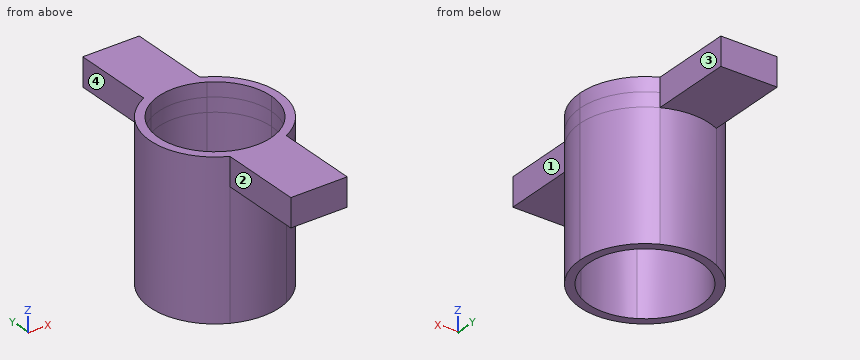
from build123d import *

# Parameters (mm, degrees)
F1_DEPTH = 10
F2_DEPTH = 1


# Not quite as in the source:
# - a feature names something its author has since deleted; it is built from what else it names


with BuildPart() as f1:
    # F0 (on Top) → F1 (new body)
    with BuildSketch(Plane.XY):
        with BuildLine():
            Line((-2, 3.4641016151), (-2, 4.1424630354))
            ThreePointArc((-2, 4.1424630354), (-4.6, 0), (-2, -4.1424630354))
            Line((-2, -4.1424630354), (-2, -3.4641016151))
            ThreePointArc((-2, -3.4641016151), (-4, 0), (-2, 3.4641016151))
        make_face()
        with BuildLine():
            ThreePointArc((-2, -4.1424630354), (0, -4.6), (2, -4.1424630354))
            Line((2, -4.1424630354), (2, -3.4641016151))
            ThreePointArc((2, -3.4641016151), (0, -4), (-2, -3.4641016151))
            Line((-2, -3.4641016151), (-2, -4.1424630354))
        make_face()
        with BuildLine():
            ThreePointArc((2, -4.1424630354), (3.8961519478, -2.4454038521), (4.6, 0))
            ThreePointArc((4.6, 0), (3.8961519478, 2.4454038521), (2, 4.1424630354))
            Line((2, 4.1424630354), (2, 3.4641016151))
            ThreePointArc((2, 3.4641016151), (3.4641016151, 2), (4, 0))
            ThreePointArc((4, 0), (3.4641016151, -2), (2, -3.4641016151))
            Line((2, -3.4641016151), (2, -4.1424630354))
        make_face()
        with BuildLine():
            Line((2, 3.4641016151), (2, 4.1424630354))
            ThreePointArc((2, 4.1424630354), (0, 4.6), (-2, 4.1424630354))
            Line((-2, 4.1424630354), (-2, 3.4641016151))
            ThreePointArc((-2, 3.4641016151), (0, 4), (2, 3.4641016151))
        make_face()
    extrude(amount=-F1_DEPTH)

    # F0 (on Top) → F2 (join, symmetric)
    with BuildSketch(Plane.XY):
        with BuildLine():
            ThreePointArc((-2, 4.1424630354), (0, 4.6), (2, 4.1424630354))
            Line((2, 4.1424630354), (2, 10))
            Line((2, 10), (-2, 10))
            Line((-2, 10), (-2, 4.1424630354))
        make_face()
        with BuildLine():
            Line((2, -10), (2, -4.1424630354))
            ThreePointArc((2, -4.1424630354), (0, -4.6), (-2, -4.1424630354))
            Line((-2, -4.1424630354), (-2, -10))
            Line((-2, -10), (2, -10))
        make_face()
        with BuildLine():
            Line((2, 3.4641016151), (2, 4.1424630354))
            ThreePointArc((2, 4.1424630354), (0, 4.6), (-2, 4.1424630354))
            Line((-2, 4.1424630354), (-2, 3.4641016151))
            ThreePointArc((-2, 3.4641016151), (0, 4), (2, 3.4641016151))
        make_face()
        with BuildLine():
            ThreePointArc((-2, -4.1424630354), (0, -4.6), (2, -4.1424630354))
            Line((2, -4.1424630354), (2, -3.4641016151))
            ThreePointArc((2, -3.4641016151), (0, -4), (-2, -3.4641016151))
            Line((-2, -3.4641016151), (-2, -4.1424630354))
        make_face()
        with BuildLine():
            Line((-2, 3.4641016151), (-2, 4.1424630354))
            ThreePointArc((-2, 4.1424630354), (-4.6, 0), (-2, -4.1424630354))
            Line((-2, -4.1424630354), (-2, -3.4641016151))
            ThreePointArc((-2, -3.4641016151), (-4, 0), (-2, 3.4641016151))
        make_face()
        with BuildLine():
            ThreePointArc((2, -4.1424630354), (3.8961519478, -2.4454038521), (4.6, 0))
            ThreePointArc((4.6, 0), (3.8961519478, 2.4454038521), (2, 4.1424630354))
            Line((2, 4.1424630354), (2, 3.4641016151))
            ThreePointArc((2, 3.4641016151), (3.4641016151, 2), (4, 0))
            ThreePointArc((4, 0), (3.4641016151, -2), (2, -3.4641016151))
            Line((2, -3.4641016151), (2, -4.1424630354))
        make_face()
    extrude(amount=F2_DEPTH, both=True)


solid = f1.part
CAD build for the part. Positions are in the model's coordinates, mm. Face numbers are marked on the shaded views. A direction names the side the tool comes from. Give positions to 0.01 mm unless a question says otherwise; leave off trailing zeros. Write each loop counter-clockwise with the first axis right and the second up, starting at its lowest first coordinate (ties: lowest second). Pieces come first, ordered by that corner, then holes. Notation, with made-up numbers: (-27, 47) -> (17, 47) arc R16 ccw to (17, 51) -> close; hole circle Ø2 at (-30.5, -19). An arc over 180 degrees is marked (long way). Return JSON: item names as keys, results as strings.
Item 1: Tool access for the marked faces 1, 2, 3 and 4: list every direction of +Z, -Z, +X, -X, +Y, -Y with a clear straight run to the whole face (end or side of a thin tool).
Answer below:
{"face 1": "+Z, -Z, +X, -Y", "face 2": "+Z, -Z, -X, -Y", "face 3": "+Z, -Z, +X, +Y", "face 4": "+Z, -Z, -X, +Y"}
Item 2: Band-saw the part on C-C (z = -5.5). List the corners of the cut face in (x, y).
Answer below:
{"outline": "circle Ø9.2 at (0, 0); hole circle Ø8 at (0, 0)"}
Item 3: Band-saw the part on A-A (y = -2). List the corners of the cut face in (x, z), then the cut area to 3 significant figures.
Answer below:
{"outline": "(-4.14, -10) -> (-3.46, -10) -> (-3.46, 1) -> (-4.14, 1) -> close; (3.46, -10) -> (4.14, -10) -> (4.14, 1) -> (3.46, 1) -> close", "area": "14.9 mm2"}
Item 4: Drill centre lines: probe 1 along X at (y, z) = (2, -6.5); probe 2 along Y at (x, z) = (3.5, -0.5); probe 3 along Y at (x, z) = (-0.75, -7). Where is each one in solid material? Low to high.
Answer below:
{"probe 1": "x = -4.14 to -3.46, 3.46 to 4.14", "probe 2": "y = -2.98 to -1.94, 1.94 to 2.98", "probe 3": "y = -4.54 to -3.93, 3.93 to 4.54"}
Item 5: Drop flat-ended pins along their axis: pin 1 (4.5 mm diameter, centred on x = -0.5, y = -8, fed in from -Z); pin 2 (2 mm diameter, centred on y = 7, z = -0.5, fed in from -X); pin 3 (5 mm diameter, centred on y = 4, z = -6.5, fed in from -X); pin 4 (3 mm diameter, centred on x = -2.5, z = -2, fed in from -Y). Give the stop position or say it passes through.
Answer below:
{"pin 1": "stops at z = -1", "pin 2": "stops at x = -2", "pin 3": "stops at x = -4.35", "pin 4": "stops at y = -10"}
Item 6: Band-saw the part on D-D (x = 3.75). List the corners of the cut face in (y, z).
Answer below:
{"outline": "(-2.66, -10) -> (-1.39, -10) -> (-1.39, 1) -> (-2.66, 1) -> close; (1.39, -10) -> (2.66, -10) -> (2.66, 1) -> (1.39, 1) -> close"}
Item 7: Band-saw the part on B-B (x = -0.5). List the corners of the cut face in (y, z), then the cut area to 3 significant figures.
Answer below:
{"outline": "(-10, -1) -> (-4.57, -1) -> (-4.57, -10) -> (-3.97, -10) -> (-3.97, 1) -> (-10, 1) -> close; (3.97, -10) -> (4.57, -10) -> (4.57, -1) -> (10, -1) -> (10, 1) -> (3.97, 1) -> close", "area": "35.0 mm2"}
